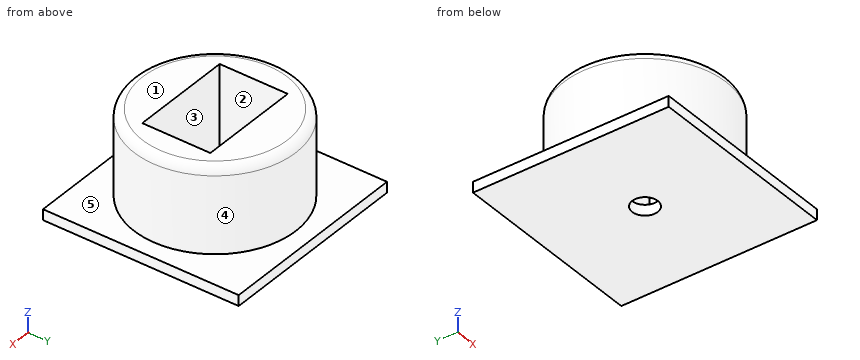
```python
from build123d import *

# Parameters (mm, degrees)
SKETCH_1_R          = 3.8
EXTRUDE_1_DEPTH     = 4
SKETCH_2_W          = 9.2
SKETCH_2_H          = 9.2
EXTRUDE_2_DEPTH     = 0.5
FILLET_1_R          = 0.4
SKETCH_4_W          = 4.8
SKETCH_4_H          = 3.2
CUT_EXTRUDE_1_DEPTH = 4
SKETCH_5_R          = 0.6
CUT_EXTRUDE_2_DEPTH = 8.636753237


with BuildPart() as part:
    # Эскиз1 → Бобышка-Вытянуть1 (new body)
    with BuildSketch(Plane.XY):
        Circle(SKETCH_1_R)
    extrude(amount=EXTRUDE_1_DEPTH)

    # Эскиз2 → Бобышка-Вытянуть2 (add)
    with BuildSketch(Plane(origin=(0, 0, 0), x_dir=(-1, 0, 0), z_dir=(0, 0, -1))):
        Rectangle(SKETCH_2_W, SKETCH_2_H)
    extrude(amount=EXTRUDE_2_DEPTH)

    # Скругление1
    fillet_1_edges = [part.edges().sort_by_distance(p)[0] for p in [
        (-3.8, 0, 4),
    ]]
    fillet(fillet_1_edges, radius=FILLET_1_R)

    # Эскиз4 → Вырез-Вытянуть1 (cut)
    with BuildSketch(Plane.XY.offset(4)):
        Rectangle(SKETCH_4_W, SKETCH_4_H)
    extrude(amount=-CUT_EXTRUDE_1_DEPTH, mode=Mode.SUBTRACT)

    # Эскиз5 → Вырез-Вытянуть2 (cut, through all)
    with BuildSketch(Plane.XY):
        Circle(SKETCH_5_R)
    extrude(amount=-CUT_EXTRUDE_2_DEPTH, mode=Mode.SUBTRACT)


solid = part.part
```
Part model, mm, in its own coordinate system. Face numbers are marked on the shaded views. A direction names the side the tool comes from. Coordinates: 2 decimals unless noted, no trailing zeros. Write each loop counter-clockwise with the first axis right and the second up, starting at its lowest first coordinate (ties: lowest second). Pieces come first, ordered by that corner, then holes.
Item 1: Slice it at A-A (y = 0). Write the cut outline in (x, z), and give its area (3 significant figures).
Item 2: Pin check, flat tips, straight feed: pin 1 (1.1 mm diameter, centred on x = 0, y = 0, fed in from -Z); pin 2 (1.6 mm diameter, centred on y = 0.5, z = 2.5, fed in from -X); pin 3 (1 mm diameter, centred on x = 1, z = 1, fed in from +Y); pin 4 (1 mm diameter, centred on x = -3, z = 1, fed in from +Y). Stop position of each tip, or through.
Item 3: Slice it at C-C (z = 3.15). Write the cut outline in (x, y), and give its area (3 significant figures).
Item 4: Mould opens along Y. For the marked faces 3, 4 and 5 say: released by +Y, released by -Y, zero draft, split by the parting line, or undercut.
Item 5: Which spindle directions (+Z, -Z, +X, -X, +Y, -Y) get a long thin tool onto all of the face, cutting with end or side? Do the marked faces 1 and 2. Say none if no direction does.
Item 6: Slice it at B-B (x = 0). Write the cut outline in (y, z), and give its area (3 significant figures).
Item 7: Probe line 1 (Y direction, x = 0, z = 3.05); line 2 (Y direction, x = 0, z = -0.3); line 3 (X direction, y = 1.25, z = 1.65). List the from-to ranges inside material, lowest first.
Results found:
1. outline: (-4.6, -0.5) - (-0.6, -0.5) - (-0.6, 0) - (-2.4, 0) - (-2.4, 4) - (-3.4, 4) arc R0.4 ccw to (-3.8, 3.6) - (-3.8, 0) - (-4.6, 0) - close; (0.6, -0.5) - (4.6, -0.5) - (4.6, 0) - (3.8, 0) - (3.8, 3.6) arc R0.4 ccw to (3.4, 4) - (2.4, 4) - (2.4, 0) - (0.6, 0) - close
1. area: 15.1 mm2
2. pin 1: passes through
2. pin 2: stops at x = -3.8
2. pin 3: stops at y = 3.77
2. pin 4: stops at y = 2.86
3. outline: circle Ø7.6 at (0, 0); hole (-2.4, -1.6) - (2.4, -1.6) - (2.4, 1.6) - (-2.4, 1.6) - close
3. area: 30.0 mm2
4. face 3: undercut
4. face 4: split by the parting line
4. face 5: zero draft
5. face 1: +Z, +X, -X, +Y, -Y
5. face 2: +Z
6. outline: (-4.6, -0.5) - (-0.6, -0.5) - (-0.6, 0) - (-1.6, 0) - (-1.6, 4) - (-3.4, 4) arc R0.4 ccw to (-3.8, 3.6) - (-3.8, 0) - (-4.6, 0) - close; (0.6, -0.5) - (4.6, -0.5) - (4.6, 0) - (3.8, 0) - (3.8, 3.6) arc R0.4 ccw to (3.4, 4) - (1.6, 4) - (1.6, 0) - (0.6, 0) - close
6. area: 21.5 mm2
7. line 1: y = -3.8 to -1.6, 1.6 to 3.8
7. line 2: y = -4.6 to -0.6, 0.6 to 4.6
7. line 3: x = -3.59 to -2.4, 2.4 to 3.59
